Build history of the part. All positions in model axes, mm. Face numbers are marked on the shaded views. A direction names the side the tool comes from. Round coordinates to 2 decimals unless told otherwise and drop trailing zeros. Write each loop counter-clockwise with the first axis right and the second up, starting at its lowest first coordinate (ties: lowest second). Pieces come first, ordered by that corner, then holes.
1) Pull direction X, two halves, no side cores. Call the marked faces 1, 2, 3 and 4: +X half, -X half, draft (parallel to the pull), parting line (faces both ways), or undercut.
2) Flat gauge pins, fed straight in: pin 1 (2 mm diameter, centred on x = -4, z = -16.5, fed in from +Y); pin 2 (1.5 mm diameter, centred on x = -10, y = 5.5, fed in from -Z); pin 3 (2 mm diameter, centred on x = 6.5, y = 2.5, fed in from -Z). Where does each tip first touch, or does it go through?
3) Saw through at B-B (x = 0.75). Write the cut outline in (y, z), plus the area to 3 significant figures.
4) Saw through at D-D (z = 6.5). Write the cut outline in (x, y), plus the area to 3 significant figures.
5) Wall check: probe 1 along X at (y, z) = (15.25, 0); probe 2 along Y at (x, z) = (-7.5, -6); probe 3 along X at (y, z) = (15, -13). Give the ranges that are in metal, low to high.
6) Which spindle directions (+Z, -Z, +X, -X, +Y, -Y) get a long thin tool onto all of the face, cutting with end or side? Do the marked faces 5 and 6. Say none if no direction does.
7) Saw through at C-C (y = 23.5). Write the cut outline in (x, z).
8) Saw through at A-A (z = 0). Write the cut outline in (x, y), plus the area to 3 significant figures.
from build123d import *

# Parameters (mm, degrees)
SKETCH1_R                       = 13.5
BOSS_EXTRUDE1_DEPTH             = 25
SKETCH2_R                       = 12.5
CUT_EXTRUDE1_DEPTH              = 24
SKETCH3_W                       = 17
SKETCH3_H                       = 8
CUT_EXTRUDE2_DEPTH              = 9
CUT_EXTRUDE3_DEPTH              = 9
SKETCH5_W                       = 2
SKETCH5_H                       = 6
BOSS_EXTRUDE2_DEPTH             = 5
BOSS_EXTRUDE2_DIRECTION_2_REACH = 41.195
SKETCH6_R                       = 1
CUT_EXTRUDE4_DEPTH              = 2


with BuildPart() as part:
    # Sketch1 → Boss-Extrude1 (new body)
    with BuildSketch(Plane(origin=(0, 0, 0), x_dir=(1, 0, 0), z_dir=(0, 1, 0))):
        with Locations(Location((0, 0, 0), (0, 0, 270))):
            Circle(SKETCH1_R)
    extrude(amount=BOSS_EXTRUDE1_DEPTH)

    # Sketch2 → Cut-Extrude1 (cut)
    with BuildSketch(Plane(origin=(0, 25, 0), x_dir=(1, 0, 0), z_dir=(0, 1, 0))):
        with Locations(Location((0, 0, 0), (0, 0, 270))):
            Circle(SKETCH2_R)
    extrude(amount=-CUT_EXTRUDE1_DEPTH, mode=Mode.SUBTRACT)

    # Sketch3 → Cut-Extrude2 (cut)
    with BuildSketch(Plane.ZY.offset(13.5)):
        with Locations((0, 6)):
            Rectangle(SKETCH3_W, SKETCH3_H)
    extrude(amount=-CUT_EXTRUDE2_DEPTH, mode=Mode.SUBTRACT)

    # Sketch4 → Cut-Extrude3 (cut)
    with BuildSketch(Plane(origin=(0, 0, -13.5), x_dir=(-1, 0, 0), z_dir=(0, 0, -1))):
        Polygon((2.5, 25), (-2.5, 25), (-2.5, 9.5), (-2.5, 6.5), (10.5, 6.5), (10.5, 9.5), (2.5, 9.5), align=None)
    extrude(amount=-CUT_EXTRUDE3_DEPTH, mode=Mode.SUBTRACT)

    # Sketch5 → Boss-Extrude2 (add)
    with BuildSketch(Plane(origin=(0, 0, -13.5), x_dir=(-1, 0, 0), z_dir=(0, 0, -1))):
        with Locations((3.5, 16.80292759)):
            Rectangle(SKETCH5_W, SKETCH5_H)
    boss_extrude2 = extrude(amount=BOSS_EXTRUDE2_DEPTH)

    # Sketch5 → Boss-Extrude2 direction 2 (add, up to next)
    with BuildSketch(Plane(origin=(0, 0, -13.5), x_dir=(-1, 0, 0), z_dir=(0, 0, -1)), mode=Mode.PRIVATE) as boss_extrude2_direction_2_sk1:
        with Locations((3.5, 16.80292759)):
            Rectangle(SKETCH5_W, SKETCH5_H)
    boss_extrude2_direction_2_tool1 = extrude(boss_extrude2_direction_2_sk1.sketch, amount=-BOSS_EXTRUDE2_DIRECTION_2_REACH, mode=Mode.PRIVATE) - part.part
    boss_extrude2_direction_2 = boss_extrude2_direction_2_tool1.solids().sort_by_distance((-3.5, 16.802928, -13.5))[0]
    add(boss_extrude2_direction_2)

    # Sketch6 → Cut-Extrude4 (cut)
    with BuildSketch(Plane(origin=(-2.5, 0, 0), x_dir=(0, 0, -1), z_dir=(1, 0, 0))):
        with Locations(Location((15.677904261, 16.72055598, 0), (0, 0, 90))):
            Circle(SKETCH6_R)
    cut_extrude4 = extrude(amount=-CUT_EXTRUDE4_DEPTH, mode=Mode.SUBTRACT)

    # Mirror1: Boss-Extrude2, Boss-Extrude2 direction 2, Cut-Extrude4 across plane
    add(boss_extrude2.mirror(Plane(origin=(0, 0, 0), x_dir=(0, 0, 1), z_dir=(1, 0, 0))))
    add(boss_extrude2_direction_2.mirror(Plane(origin=(0, 0, 0), x_dir=(0, 0, 1), z_dir=(1, 0, 0))))
    add(cut_extrude4.mirror(Plane(origin=(0, 0, 0), x_dir=(0, 0, 1), z_dir=(1, 0, 0))), mode=Mode.SUBTRACT)


solid = part.part
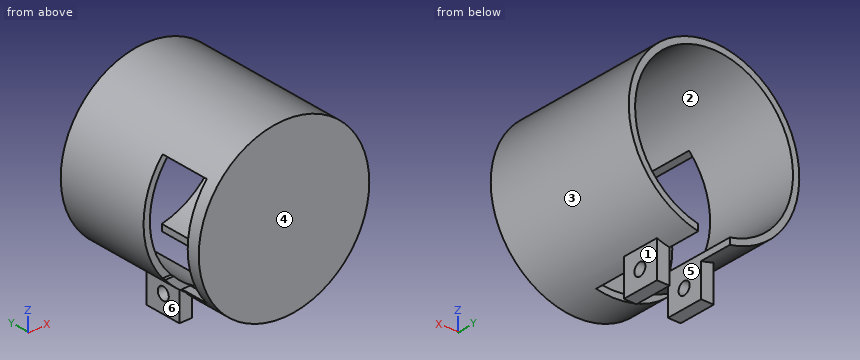
Evaluation:
1. face 1: +X half
1. face 2: undercut
1. face 3: parting line
1. face 4: draft
2. pin 1: stops at y = 19.8
2. pin 2: stops at z = -9.83
2. pin 3: stops at z = -12.33
3. outline: (0, -13.48) - (6.5, -13.48) - (6.5, -12.48) - (1, -12.48) - (1, 12.48) - (25, 12.48) - (25, 13.48) - (0, 13.48) - close
3. area: 56.5 mm2
4. outline: (-11.83, 0) - (11.83, 0) - (11.83, 25) - (10.68, 25) - (10.68, 1) - (-10.68, 1) - (-10.68, 2) - (-11.83, 2) - close; (-11.83, 10) - (-10.68, 10) - (-10.68, 25) - (-11.83, 25) - close
4. area: 69.9 mm2
5. probe 1: x = -13.5 to -12.5, 12.5 to 13.5
5. probe 2: y = 0 to 1
5. probe 3: x = -4.5 to -2.5, 2.5 to 4.5
6. face 5: -Z, +Y
6. face 6: -Z, -X, +Y, -Y
7. outline: (-2.5, -13.27) - (-2.5, -12.25) arc R12.5 cw (long way) to (2.5, -12.25) - (2.5, -13.27) arc R13.5 ccw (long way) to start
8. outline: (-13.5, 0) - (13.5, 0) - (13.5, 25) - (12.5, 25) - (12.5, 1) - (-12.5, 1) - (-12.5, 2) - (-13.5, 2) - close; (-13.5, 10) - (-12.5, 10) - (-12.5, 25) - (-13.5, 25) - close
8. area: 67.0 mm2
